```python
from build123d import *

# Parameters (mm, degrees)
SKETCH3_W              = 455.295
SKETCH3_H              = 277.368
BOSS_EXTRUDE1_DEPTH    = 1.5875
CUT_EXTRUDE1_DEPTH     = 25.4
SKETCH8_W              = 40.894
SKETCH8_H              = 48.26
CUT_EXTRUDE2_DEPTH     = 25.4
F_10_CLEARANCE_HOLE1_D = 4.9784
F_10_CLEARANCE_HOLE2_D = 4.9784


with BuildPart() as part:
    # Sketch3 → Boss-Extrude1 (new, symmetric)
    with BuildSketch(Plane.XY):
        Rectangle(SKETCH3_W, SKETCH3_H)
    extrude(amount=BOSS_EXTRUDE1_DEPTH, both=True)

    # Sketch4 → Cut-Extrude1 (cut)
    with BuildSketch(Plane.XY.offset(1.5875)):
        with BuildLine():
            Line((-161.29, 54.991001016), (-143.51, 54.991001016))
            ThreePointArc((-143.51, 54.991001016), (-139.917897552, 53.503103464), (-138.43, 49.911001016))
            Line((-138.43, 49.911001016), (-138.43, 9.271001016))
            ThreePointArc((-138.43, 9.271001016), (-139.917897552, 5.678898568), (-143.51, 4.191001016))
            Line((-143.51, 4.191001016), (-161.29, 4.191001016))
            ThreePointArc((-161.29, 4.191001016), (-164.882102448, 5.678898568), (-166.37, 9.271001016))
            Line((-166.37, 9.271001016), (-166.37, 49.911001016))
            ThreePointArc((-166.37, 49.911001016), (-164.882102448, 53.503103464), (-161.29, 54.991001016))
        make_face()
        with BuildLine():
            Line((-8.89, 54.991001016), (8.89, 54.991001016))
            ThreePointArc((8.89, 54.991001016), (12.482102448, 53.503103464), (13.97, 49.911001016))
            Line((13.97, 49.911001016), (13.97, 9.271001016))
            ThreePointArc((13.97, 9.271001016), (12.482102448, 5.678898568), (8.89, 4.191001016))
            Line((8.89, 4.191001016), (-8.89, 4.191001016))
            ThreePointArc((-8.89, 4.191001016), (-12.482102448, 5.678898568), (-13.97, 9.271001016))
            Line((-13.97, 9.271001016), (-13.97, 49.911001016))
            ThreePointArc((-13.97, 49.911001016), (-12.482102448, 53.503103464), (-8.89, 54.991001016))
        make_face()
        with BuildLine():
            Line((67.31, 54.991001016), (85.09, 54.991001016))
            ThreePointArc((85.09, 54.991001016), (88.682102448, 53.503103464), (90.17, 49.911001016))
            Line((90.17, 49.911001016), (90.17, 9.271001016))
            ThreePointArc((90.17, 9.271001016), (88.682102448, 5.678898568), (85.09, 4.191001016))
            Line((85.09, 4.191001016), (67.31, 4.191001016))
            ThreePointArc((67.31, 4.191001016), (63.717897552, 5.678898568), (62.23, 9.271001016))
            Line((62.23, 9.271001016), (62.23, 49.911001016))
            ThreePointArc((62.23, 49.911001016), (63.717897552, 53.503103464), (67.31, 54.991001016))
        make_face()
        with BuildLine():
            Line((143.51, 54.991001016), (161.29, 54.991001016))
            ThreePointArc((161.29, 54.991001016), (164.882102448, 53.503103464), (166.37, 49.911001016))
            Line((166.37, 49.911001016), (166.37, 9.271001016))
            ThreePointArc((166.37, 9.271001016), (164.882102448, 5.678898568), (161.29, 4.191001016))
            Line((161.29, 4.191001016), (143.51, 4.191001016))
            ThreePointArc((143.51, 4.191001016), (139.917897552, 5.678898568), (138.43, 9.271001016))
            Line((138.43, 9.271001016), (138.43, 49.911001016))
            ThreePointArc((138.43, 49.911001016), (139.917897552, 53.503103464), (143.51, 54.991001016))
        make_face()
        with BuildLine():
            Line((-85.09, 54.991001016), (-67.31, 54.991001016))
            ThreePointArc((-67.31, 54.991001016), (-63.717897552, 53.503103464), (-62.23, 49.911001016))
            Line((-62.23, 49.911001016), (-62.23, 9.271001016))
            ThreePointArc((-62.23, 9.271001016), (-63.717897552, 5.678898568), (-67.31, 4.191001016))
            Line((-67.31, 4.191001016), (-85.09, 4.191001016))
            ThreePointArc((-85.09, 4.191001016), (-88.682102448, 5.678898568), (-90.17, 9.271001016))
            Line((-90.17, 9.271001016), (-90.17, 49.911001016))
            ThreePointArc((-90.17, 49.911001016), (-88.682102448, 53.503103464), (-85.09, 54.991001016))
        make_face()
    extrude(amount=-CUT_EXTRUDE1_DEPTH, mode=Mode.SUBTRACT)

    # Sketch8 → Cut-Extrude2 (cut)
    with BuildSketch(Plane.XY.offset(1.5875)):
        with Locations((-207.2005, -114.554)):
            Rectangle(SKETCH8_W, SKETCH8_H)
        with Locations((207.2005, -114.554)):
            Rectangle(SKETCH8_W, SKETCH8_H)
    extrude(amount=-CUT_EXTRUDE2_DEPTH, mode=Mode.SUBTRACT)

    # #10 Clearance Hole1 (through all)
    with Locations(Plane.XY.offset(1.5875)):
        with Locations((208.5975, 125.984), (208.5975, 51.816), (208.5975, -70.866), (-208.5975, -70.866), (-208.5975, 51.816), (-208.5975, 125.984)):
            Hole(F_10_CLEARANCE_HOLE1_D / 2)

    # #10 Clearance Hole2 (through all)
    with Locations(Plane(origin=(0, 0, -1.5875), x_dir=(-1, 0, 0), z_dir=(0, 0, -1))):
        with Locations((0, 59.7535)):
            Hole(F_10_CLEARANCE_HOLE2_D / 2)


solid = part.part
```
The listing builds one solid part. Answer for the finished solid, in the listing's coordinates (mm). Coordinates: 2 decimals unless noted, no trailing zeros. Use a Markdown table: item, result. Add a question column.
1) Given pin 1 (3 mm diameter, centred on x = -208.6, y = 51.82, fed in from -Z); pin 2 (1 mm diameter, centred on y = -123.5, z = -0.5, fed in from +X); pin 3 (1 mm diameter, centred on x = -204, z = 0.5, fed in from -Y), each flat-ended and moving along its own axis, determine where each tip first touches the part or whether it passes through.
2) The part is cut by section A-A, the plane z = -1. State how many separate pieces and enclosed holes the cut face has, and give its area (3 significant figures).
3) Find the intervals of material crossed by line 1 (X direction, y = 37, z = 0.45); line 2 (Y direction, x = 67, z = -1.3); line 3 (Y direction, x = 1.5, z = -0.3), in increasing order.
Here are the results:
| question | item | result |
|---|---|---|
| 1 | pin 1 | passes through |
| 1 | pin 2 | stops at x = 186.75 |
| 1 | pin 3 | stops at y = -90.42 |
| 2 | separate pieces | 1 |
| 2 | enclosed holes | 12 |
| 2 | area | 115,000 mm^2 |
| 3 | line 1 | x = -227.65 to -166.37, -138.43 to -90.17, -62.23 to -13.97, 13.97 to 62.23, 90.17 to 138.43, 166.37 to 227.65 |
| 3 | line 2 | y = -138.68 to 4.2, 54.98 to 138.68 |
| 3 | line 3 | y = -138.68 to 4.19, 54.99 to 57.77, 61.74 to 138.68 |
